from build123d import *

# Parameters (mm, degrees)
EXTRUDE_START       = 74.5
SKETCH_4_R          = 2
EXTRUDE_1_DEPTH     = 6
SKETCH_5_W          = 40
SKETCH_5_H          = 34
SKETCH_5_R          = 2
EXTRUDE_2_DEPTH     = 7
CUT_EXTRUDE_START   = -21.5
SKETCH_6_R          = 4
CUT_EXTRUDE_1_DEPTH = 3
EXTRUDE_START_2     = 40.5
SKETCH_7_R          = 4.1
EXTRUDE_3_DEPTH     = 7
SKETCH_8_R          = 4.9
CUT_EXTRUDE_2_DEPTH = 0.9
EXTRUDE_START_3     = 2
EXTRUDE_4_DEPTH     = 6
EXTRUDE_5_DEPTH     = 6
SKETCH_13_W         = 30
SKETCH_13_H         = 25
EXTRUDE_6_DEPTH     = 7


with BuildPart() as part:
    # 草图4 → 凸台-拉伸1 (new body)
    with BuildSketch(Plane(origin=(0, 0, 0), x_dir=(1, 0, 0), z_dir=(0, 1, 0)).offset(EXTRUDE_START)):
        with BuildLine():
            Line((-28, 28.5), (28, 28.5))
            Line((28, 28.5), (28, 2.5))
            ThreePointArc((28, 2.5), (27.121320344, 0.378679656), (25, -0.5))
            Line((25, -0.5), (21, -0.5))
            Line((21, -0.5), (21, 21.5))
            Line((21, 21.5), (-21, 21.5))
            Line((-21, 21.5), (-21, -0.5))
            Line((-21, -0.5), (-25, -0.5))
            ThreePointArc((-25, -0.5), (-27.121320344, 0.378679656), (-28, 2.5))
            Line((-28, 2.5), (-28, 28.5))
        make_face()
        with Locations(Location((-24.2, 14.9, 0), (0, 0, 90))):
            Circle(SKETCH_4_R, mode=Mode.SUBTRACT)
        with Locations(Location((-24.2, 5.1, 0), (0, 0, 90))):
            Circle(SKETCH_4_R, mode=Mode.SUBTRACT)
        with Locations(Location((24.2, 14.9, 0), (0, 0, 90))):
            Circle(SKETCH_4_R, mode=Mode.SUBTRACT)
        with Locations(Location((24.2, 5.1, 0), (0, 0, 90))):
            Circle(SKETCH_4_R, mode=Mode.SUBTRACT)
    extrude(amount=EXTRUDE_1_DEPTH)

    # 草图5 → 凸台-拉伸2 (add)
    with BuildSketch(Plane(origin=(0, 0, -28.5), x_dir=(-1, 0, 0), z_dir=(0, 0, -1))):
        with Locations((0, 57.5)):
            Rectangle(SKETCH_5_W, SKETCH_5_H)
        with Locations((-10, 72)):
            Circle(SKETCH_5_R, mode=Mode.SUBTRACT)
        with Locations(Location((10, 72, 0), (0, 0, 180))):
            Circle(SKETCH_5_R, mode=Mode.SUBTRACT)
        with Locations((10, 57)):
            Circle(SKETCH_5_R, mode=Mode.SUBTRACT)
        with Locations(Location((-10, 57, 0), (0, 0, 180))):
            Circle(SKETCH_5_R, mode=Mode.SUBTRACT)
    extrude(amount=-EXTRUDE_2_DEPTH)

    # 草图6 → 切除-拉伸1 (cut)
    with BuildSketch(Plane.XY.offset(CUT_EXTRUDE_START)):
        with Locations((-10, 72)):
            Circle(SKETCH_6_R)
        with Locations((10, 72)):
            Circle(SKETCH_6_R)
        with Locations((-10, 57)):
            Circle(SKETCH_6_R)
        with Locations((10, 57)):
            Circle(SKETCH_6_R)
    extrude(amount=-CUT_EXTRUDE_1_DEPTH, mode=Mode.SUBTRACT)

    # 草图7 → 凸台-拉伸3 (add)
    with BuildSketch(Plane(origin=(0, 0, 0), x_dir=(1, 0, 0), z_dir=(0, 1, 0)).offset(EXTRUDE_START_2)):
        with BuildLine():
            Line((20, 21.5), (-20, 21.5))
            Line((-20, 21.5), (-20, 1.5))
            ThreePointArc((-20, 1.5), (-19.121320344, -0.621320344), (-17, -1.5))
            Line((-17, -1.5), (17, -1.5))
            ThreePointArc((17, -1.5), (19.121320344, -0.621320344), (20, 1.5))
            Line((20, 1.5), (20, 21.5))
        make_face()
        with Locations(Location((10, 10, 0), (0, 0, 90))):
            Circle(SKETCH_7_R, mode=Mode.SUBTRACT)
    extrude(amount=EXTRUDE_3_DEPTH)

    # 草图8 → 切除-拉伸2 (cut)
    with BuildSketch(Plane.XZ.offset(-40.5)):
        with Locations(Location((10, -10, 0), (0, 0, 270))):
            Circle(SKETCH_8_R)
    extrude(amount=-CUT_EXTRUDE_2_DEPTH, mode=Mode.SUBTRACT)

    # 草图10 → 凸台-拉伸4 (add)
    with BuildSketch(Plane(origin=(20, 0, 0), x_dir=(0, 0, -1), z_dir=(1, 0, 0)).offset(EXTRUDE_START_3)):
        Polygon((28.5, 49.5), (28.5, 74.5), (17, 74.5), (21.5, 49.5), align=None)
    extrude(amount=EXTRUDE_4_DEPTH)

    # 草图12 → 凸台-拉伸5 (add)
    with BuildSketch(Plane.ZY.offset(20).offset(EXTRUDE_START_3)):
        Polygon((-21.5, 49.5), (-28.5, 49.5), (-28.5, 74.5), (-17, 74.5), align=None)
    extrude(amount=EXTRUDE_5_DEPTH)

    # 草图13 → 凸台-拉伸6 (add)
    with BuildSketch(Plane(origin=(0, 0, -28.5), x_dir=(-1, 0, 0), z_dir=(0, 0, -1))):
        with BuildLine():
            Line((28, 80.5), (-28, 80.5))
            Line((-28, 80.5), (-28, 45.5))
            ThreePointArc((-28, 45.5), (-26.535533906, 41.964466094), (-23, 40.5))
            Line((-23, 40.5), (23, 40.5))
            ThreePointArc((23, 40.5), (26.535533906, 41.964466094), (28, 45.5))
            Line((28, 45.5), (28, 80.5))
        make_face()
        with Locations((0, 65)):
            Rectangle(SKETCH_13_W, SKETCH_13_H, mode=Mode.SUBTRACT)
    extrude(amount=-EXTRUDE_6_DEPTH)


solid = part.part
Read the model definition and answer for the solid it produces. Units are mm, in the model's axes. A direction names the side the tool comes from. Round coordinates to 2 decimals unless told otherwise and drop trailing zeros. Write each loop counter-clockwise with the first axis right and the second up, starting at its lowest first coordinate (ties: lowest second). Pieces come first, ordered by that corner, then holes.
1. Determine the mould class of faces 4 (the face through (-24, 74.5, -8)), 5 (the face through (-23.434, 77.458, -16.747)), 6 (the face through (0, 65, -21.5)) for opening direction Z: pulls with the +Z half, pulls with the -Z half, needs draft (parallel to the pull), parting line crosses it, or undercut.
2. The part is cut by section C-C, the plane x = -10. Determine the outline of the cut face in (y, z).
3. The part is cut by section D-D, the plane y = 57. Determine the outline of the cut face in (x, z).
4. Which of the six approach directions +Z, -Z, +X, -X, +Y, -Y give full straight-line access (tool end or side, diameter ignored) to faces 1 (the face through (0, 47.5, -10)), 2 (the face through (9.133, 53.095, -22.979)), 3 (the face through (-21, 77, -11))?
5. Given pin 1 Ø3 at (x, y) = (0, 48) entering from +Z; pin 2 Ø5 at (x, y) = (-10, 72) entering from +Z; pin 3 Ø11.5 at (x, z) = (10, -10) entering from +Y; pin 4 Ø8 at (x, y) = (-12, 75) entering from +Z, each flat-ended and moving along its own axis, determine where each tip first touches the part or whether it passes through.
6. The part is cut by section A-A, the plane z = -23.5. Determine the outline of the cut face in (x, y), then the cut area to 3 significant figures.
7. Straight lines are drawn through the part: L1, parallel to Z at x = 24.2, y = 78; L2, parallel to Y at x = -10, z = -27.55; L3, parallel to Z at x = -18, y = 66. For each, find the intervals that lie inside material, in ascending order.
8. The part is cut by section B-B, the plane x = 10. State how many separate pieces and enclosed holes the cut face has, then the cut area to 3 significant figures.
Values:
1. face 4: needs draft
1. face 5: undercut
1. face 6: pulls with the +Z half
2. outline: (40.5, -28.5) - (55, -28.5) - (55, -24.5) - (53, -24.5) - (53, -21.5) - (47.5, -21.5) - (47.5, 1.5) - (40.5, 1.5) - close; (59, -28.5) - (70, -28.5) - (70, -24.5) - (68, -24.5) - (68, -21.5) - (61, -21.5) - (61, -24.5) - (59, -24.5) - close; (74, -28.5) - (80.5, -28.5) - (80.5, -21.5) - (76, -21.5) - (76, -24.5) - (74, -24.5) - close
3. outline: (-28, -28.5) - (-12, -28.5) - (-12, -24.5) - (-14, -24.5) - (-14, -21.5) - (-22, -21.5) - (-22, -20.15) - (-28, -20.15) - close; (-8, -28.5) - (8, -28.5) - (8, -24.5) - (6, -24.5) - (6, -21.5) - (-6, -21.5) - (-6, -24.5) - (-8, -24.5) - close; (12, -28.5) - (28, -28.5) - (28, -20.15) - (22, -20.15) - (22, -21.5) - (14, -21.5) - (14, -24.5) - (12, -24.5) - close
4. face 1: +Z, +X, -X, +Y
4. face 2: +Z
4. face 3: +Z, +Y, -Y
5. pin 1: stops at z = 1.5
5. pin 2: stops at z = -24.5
5. pin 3: stops at y = 47.5
5. pin 4: stops at z = -21.5
6. outline: (-28, 45.5) arc R5 ccw to (-23, 40.5) - (23, 40.5) arc R5 ccw to (28, 45.5) - (28, 80.5) - (-28, 80.5) - close; hole circle Ø8 at (-10, 57); hole circle Ø8 at (-10, 72); hole circle Ø8 at (10, 57); hole circle Ø8 at (10, 72)
6. area: 2,030 mm2
7. L1: z = -28.5 to -16.9, -12.9 to -7.1, -3.1 to 0.5
7. L2: y = 40.5 to 55, 59 to 70, 74 to 80.5
7. L3: z = -28.5 to -21.5
8. separate pieces: 4
8. enclosed holes: 0
8. area: 302 mm2
